from build123d import *

# Parameters (mm, degrees)
F1_DEPTH  = 60
F2_W      = 50
F2_H      = 13
F3_DEPTH  = 13
F4_W      = 50
F4_H      = 13
F5_DEPTH  = 13
F6_R      = 29.99999
F7_R      = 10
F9_DEPTH  = 20
F8_R      = 10
F10_DEPTH = 60


# Not quite as in the source:
# - a fillet or chamfer is up to 0.001 mm smaller than in the source, because OpenCascade refuses the exact size


with BuildPart() as f1:
    # F0 (on Front) → F1 (new body)
    with BuildSketch(Plane.XZ):
        Polygon((-44.2382382879, 60), (-44.2382382879, 0), (20.7617617121, 0), (20.7617617121, 7), (70.7617617121, 7), (70.7617617121, 27), (5.7617617121, 27), (5.7617617121, 60), align=None)
    extrude(amount=F1_DEPTH)

    # F2 (on face) → F3 (join)
    with BuildSketch(Plane.XY.offset(60)):
        with Locations((-19.2382382879, -6.5)):
            Rectangle(F2_W, F2_H)
    extrude(amount=F3_DEPTH)

    # F4 (on face) → F5 (join)
    with BuildSketch(Plane.XY.offset(60)):
        with Locations((-19.2382382879, -53.5)):
            Rectangle(F4_W, F4_H)
    extrude(amount=F5_DEPTH)

    # F6 (radius 30 in the source; OpenCascade refuses exactly that, so slightly less here)
    f6_edges = [f1.edges().sort_by_distance(p)[0] for p in [
        (70.761762, -60, 17),
        (70.761762, 0, 17),
    ]]
    fillet(f6_edges, radius=F6_R)

    # F7 (on face) → F9 (cut)
    with BuildSketch(Plane.XY.offset(27)):
        with Locations((40.7617617121, -30)):
            Circle(F7_R)
    extrude(amount=-F9_DEPTH, mode=Mode.SUBTRACT)

    # F8 (on face) → F10 (cut)
    with BuildSketch(Plane.XY.offset(60)):
        with Locations((-19.2382382879, -30)):
            Circle(F8_R)
    extrude(amount=-F10_DEPTH, mode=Mode.SUBTRACT)


solid = f1.part
Geometry: final body of the model. Coordinates: model frame, mm. A direction names the side the tool comes from. Round coordinates to 2 decimals unless told otherwise and drop trailing zeros. Loops run counter-clockwise (first coordinate to the right, second up) from the corner with the lowest first, then second, coordinate; pieces in that order, holes last. Notation, with made-up numbers: M 37,47.5 L 80,47.5 A25 cw 80,77.5 Z; hole C 40,12 d11. An arc over 180 degrees is marked long. One line per question, with ' | ' between items.
(1) Access query for faces 1 (the flat face through (-20, -53, 73)), 2 (the flat face through (51, -30, 7)), 3 (the flat face through (31, -36, 27)), 4 (the flat face through (-20, -13, 66)). Directions: +Z, -Z, +X, -X, +Y, -Y. A direction counts if a zero-diameter tool reaches every point of the face in a straight line with its end or side. Return the directions, or none.
Check result:
face 1: +Z, +X, -X, +Y, -Y | face 2: -Z, +X, +Y, -Y | face 3: +Z, +X, +Y, -Y | face 4: +Z, +X, -X
(2) Pull-direction query (Y, two-part tool) for faces 5 (the cylindrical face through (-14.62, -38.87, 30.42)), 6 (the flat face through (5.762, -30, 50)), 7 (the cylindrical face through (61.74, -51.445, 17.14)); classes: +Y half, -Y half, draft (parallel to the pull), parting line (faces both ways), or undercut.
Check result:
face 5: undercut | face 6: draft | face 7: -Y half
(3) Cut plane D-D on x = 17. Return the cut outline in (y, z), plus the area to 3 significant figures.
Check result:
outline: M -60,0 L 0,0 L 0,27 L -60,27 Z | area: 1,620 mm2
(4) Cut plane A-A on z = 38.5. Return the cut outline in (x, y), plus the area to 3 significant figures.
Check result:
outline: M -44.24,-60 L 5.76,-60 L 5.76,0 L -44.24,0 Z; hole C -19.24,-30 d20 | area: 2,690 mm2
(5) Contact query for flat-ended pins moving along their axis: P1, Ø14, axis at y = -44.5, z = 59.5, coming from the +X side; P2, Ø3.5, axis at y = -28, z = 3.5, coming from the +X side; P3, Ø12, axis at x = 19.5, y = -18, coming from the +Z side. Output: stop coordinate, or through.
Check result:
P1: stops at x = 5.76 | P2: stops at x = 20.76 | P3: stops at z = 27
(6) Material intervals for line 1 along X through (y, z) = (-29.5, 30); line 2 along Z through (x, y) = (7, -31.5); line 3 along X through (y, z) = (-50.5, 61.5), sorted ascending. Write a range as from..to.
Check result:
line 1: x = -44.24..-29.23, -9.25..5.76 | line 2: z = 0..27 | line 3: x = -44.24..5.76
(7) Cut plane B-B on x = 44.5. Return the cut outline in (y, z) (3 decimals), plus the area to 3 significant figures.
Check result:
outline: M -59.766,7 L -39.275,7 L -39.275,27 L -59.766,27 Z; M -20.725,7 L -0.234,7 L -0.234,27 L -20.725,27 Z | area: 820 mm2
(8) Cut plane C-C on y = -38. Return the cut outline in (x, z).
Check result:
outline: M -44.24,0 L -25.24,0 L -25.24,60 L -44.24,60 Z; M -13.24,0 L 20.76,0 L 20.76,7 L 34.76,7 L 34.76,27 L 5.76,27 L 5.76,60 L -13.24,60 Z; M 46.76,7 L 69.68,7 L 69.68,27 L 46.76,27 Z
